Design review of the part shown in the three views and the two pictorial views. Dimensions are in mm from the part's minimum x, y and z. Coordinates: 2 decimals unless noted, no trailing zeros. Write each loop counter-clockwise with the first axis right and the second up, starting at its lowest first coordinate (ties: lowest second). Pieces come first, ordered by that corner, then holes. Notation, with made-up numbers: (60, 22.5) - (108, 22.5) arc R24 ccw to (108, 46.5) - close; hole circle Ø3 at (-37, -7.75). An arc over 180 degrees is marked (long way). Write each question's results on one line, items separated by ' | '.
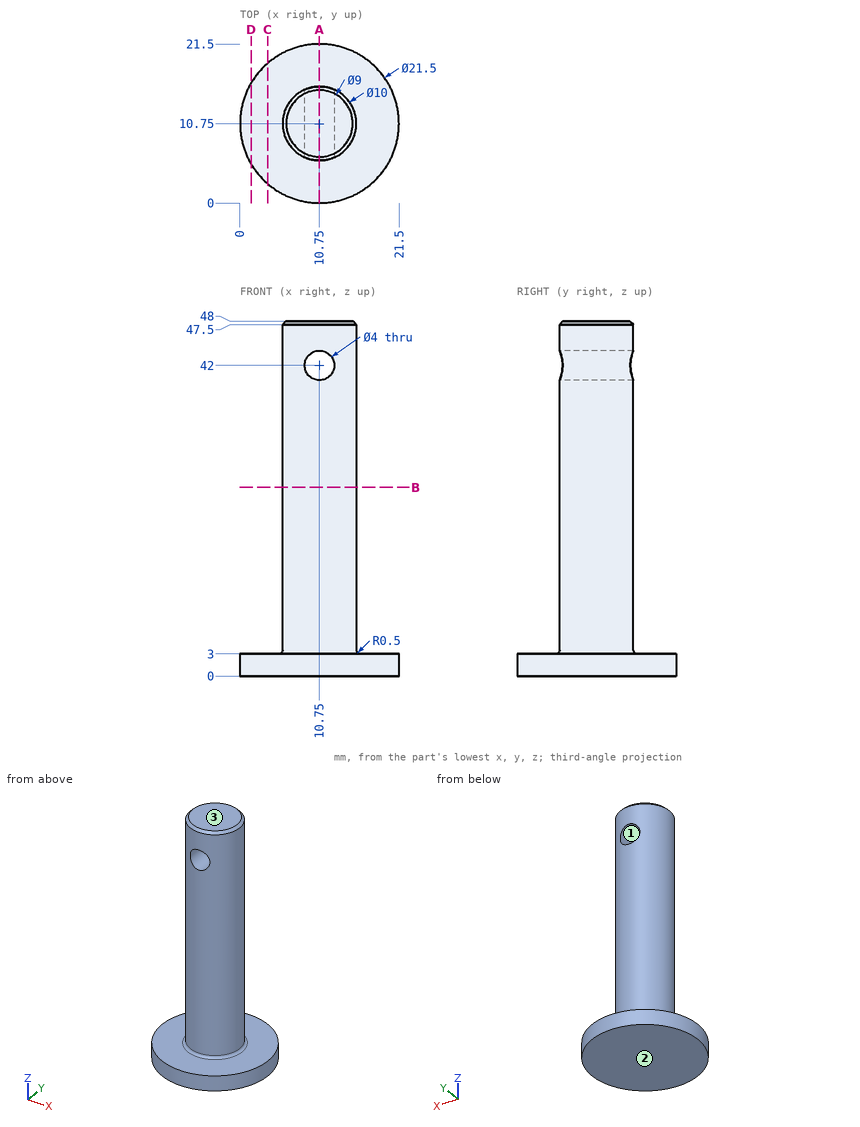
Q1. Take a section at B-B on z = 25.5. State the section outline as (x, y) points.
Results found:
outline: circle Ø10 at (10.75, 10.75)
Q2. Take a section at C-C on x = 3.75. State the section outline as (y, z) points.
Results found:
outline: (2.59, 0) - (18.91, 0) - (18.91, 3) - (2.59, 3) - close
Q3. Wall thickness on line 1 along Z through (x, y) = (10.75, 12); line 2 along X through (y, z) = (13.75, 42); line 3 along Z through (x, y) = (18.5, 14): over which ranges is each line inside the solid? List them lowest first. Write a range as from..to.
Results found:
line 1: 0..40, 44..48 | line 2: 6.75..8.75, 12.75..14.75 | line 3: 0..3
Q4. Mouldability with a two-part tool opening along Z and no side actions: class the marked faces 1, 2 and 3 as pulls with the +Z half, pulls with the -Z half, needs draft (parallel to the pull), parting line crosses it, or undercut.
Results found:
face 1: undercut | face 2: pulls with the -Z half | face 3: pulls with the +Z half
Q5. Take a section at A-A on x = 10.75. State the section outline as (y, z) points, plus the area to 3 significant figures.
Results found:
outline: (0, 0) - (21.5, 0) - (21.5, 3) - (16.25, 3) arc R0.5 cw to (15.75, 3.5) - (15.75, 40) - (5.75, 40) - (5.75, 3.5) arc R0.5 cw to (5.25, 3) - (0, 3) - close; (5.75, 44) - (15.75, 44) - (15.75, 47.5) - (15.25, 48) - (6.25, 48) - (5.75, 47.5) - close | area: 474 mm2
Q6. For pin 1 (1.5 mm diameter, centred on y = 13.5, z = 42, fed in from +X); pin 2 (2 mm diameter, centred on y = 12, z = 27.5, fed in from +X); pin 3 (1.5 mm diameter, centred on x = 5.5, y = 18, fed in from +Z), all flat-tipped, find the tip position at first contact; note any pin that passes through.
Results found:
pin 1: x = 15.33 | pin 2: x = 15.74 | pin 3: z = 3
Q7. Take a section at D-D on x = 1.5. State the section outline as (y, z) points, plus the area to 3 significant figures.
Results found:
outline: (5.27, 0) - (16.23, 0) - (16.23, 3) - (5.27, 3) - close | area: 32.9 mm2
